The listing builds one solid part. Answer for the finished solid, in the listing's coordinates (mm). A direction names the side the tool comes from. Give positions to 0.01 mm unless a question says otherwise; leave off trailing zeros. Order: outer loops, then holes, each group sorted by start corner. A loop starts at its lowest first (then second) coordinate and runs counter-clockwise, first axis right, second up. Notation, with made-up numbers: (61.5, 72.25) - (117.5, 72.25) arc R28 ccw to (117.5, 97.25) - close; hole circle Ø2 at (7.5, 55.5). An arc over 180 degrees is marked (long way). Answer as CSV lines item,"result". Start each with the question number.
1. Which of the six approach directions +Z, -Z, +X, -X, +Y, -Y give full straight-line access (tool end or side, diameter ignored) to faces 1 (the flat face through (-9, -8, 110.5)), 2 (the flat face through (-21, -8, 123)), 3 (the flat face through (-9, -18, 102)), 4 (the flat face through (24, -18, 123)), 5 (the flat face through (-41, -18, 123))?
2. Section A-A on x = 1 is taken. Give the vertices of the cut face in (y, z).
3. Section C-C on y = -15.75 is taken. Give the vertices of the cut face in (x, z), and give its area (3 significant figures).
4. Flat-ended cylindrical pins translate along their axes: pin 1 (2.5 mm diameter, centred on x = -9, y = -9, fed in from +Z); pin 2 (4 mm diameter, centred on x = -8, y = -17, fed in from +Z); pin 3 (6.5 mm diameter, centred on y = -7.5, z = 122.5, fed in from -X). Find the tip coordinate at first contact, or state that the pin passes through.
5. Consider line 1 along Y through (x, z) = (-28, 120); line 2 along Z through (x, y) = (-27, -19); line 3 along X through (y, z) = (-8.5, 120). Determine where each line is inside the solid, lowest interval first. Write a range as [from, to].
6. Section D-D on z = 105.5 is taken. Give the vertices of the cut face in (x, y), and give its area (3 significant figures).
7. Section B-B on z = 125.5 is taken. Give the vertices of the cut face in (x, y).
from build123d import *

# Parameters (mm, degrees)
SKETCH1_W        = 75
SKETCH1_H        = 52
ESP32_PCB_DEPTH  = 1.6
SKETCH2_W        = 25
SKETCH2_H        = 25
GNSS_PATCH_DEPTH = 8
SKETCH3_W        = 65
SKETCH3_H        = 42
LIPO_DEPTH       = 8


with BuildPart() as part:
    # Sketch1 → ESP32 PCB (new body)
    with BuildSketch(Plane(origin=(0, -14, 0), x_dir=(1, 0, 0), z_dir=(0, 1, 0))):
        with Locations((-8.5, -123)):
            Rectangle(SKETCH1_W, SKETCH1_H)
    extrude(amount=ESP32_PCB_DEPTH)

    # Sketch2 → GNSS Patch (add)
    with BuildSketch(Plane(origin=(0, -12.4, 0), x_dir=(1, 0, 0), z_dir=(0, 1, 0))):
        with Locations((-8.5, -123)):
            Rectangle(SKETCH2_W, SKETCH2_H)
    extrude(amount=GNSS_PATCH_DEPTH)

    # Sketch3 → LiPo (add)
    with BuildSketch(Plane(origin=(0, -22, 0), x_dir=(1, 0, 0), z_dir=(0, 1, 0))):
        with Locations((-8.5, -123)):
            Rectangle(SKETCH3_W, SKETCH3_H)
    extrude(amount=LIPO_DEPTH)


solid = part.part
Checks:
1,face 1,"-Z, +X, -X, +Y"
1,face 2,"+Z, -Z, -X, +Y"
1,face 3,"-Z, +X, -X, -Y"
1,face 4,"+Z, -Z, +X, -Y"
1,face 5,"+Z, -Z, -X, -Y"
2,outline,"(-22, 102) - (-14, 102) - (-14, 97) - (-12.4, 97) - (-12.4, 110.5) - (-4.4, 110.5) - (-4.4, 135.5) - (-12.4, 135.5) - (-12.4, 149) - (-14, 149) - (-14, 144) - (-22, 144) - close"
3,outline,"(-41, 102) - (24, 102) - (24, 144) - (-41, 144) - close"
3,area,"2,730 mm²"
4,pin 1,"stops at z = 135.5"
4,pin 2,"stops at z = 144"
4,pin 3,"stops at x = -21"
5,line 1,"y = [-22, -12.4]"
5,line 2,"z = [102, 144]"
5,line 3,"x = [-21, 4]"
6,outline,"(-46, -14) - (-41, -14) - (-41, -22) - (24, -22) - (24, -14) - (29, -14) - (29, -12.4) - (-46, -12.4) - close"
6,area,"640 mm²"
7,outline,"(-46, -14) - (-41, -14) - (-41, -22) - (24, -22) - (24, -14) - (29, -14) - (29, -12.4) - (4, -12.4) - (4, -4.4) - (-21, -4.4) - (-21, -12.4) - (-46, -12.4) - close"
